```python
from build123d import *

# Parameters (mm, degrees)
SKETCH1_W                    = 104.78
SKETCH1_H                    = 53.63
BOSS_EXTRUDE1_DEPTH          = 6.35
F_0_257_DIAMETER_HOLE1_D     = 6.5278
F_30_0_1285_DIAMETER_HOLE1_D = 3.2639
FILLET1_R                    = 5


with BuildPart() as part:
    # Sketch1 → Boss-Extrude1 (new body)
    with BuildSketch(Plane(origin=(0, 0, 0), x_dir=(1, 0, 0), z_dir=(0, 1, 0))):
        with Locations((52.39, 26.815)):
            Rectangle(SKETCH1_W, SKETCH1_H)
    extrude(amount=BOSS_EXTRUDE1_DEPTH)

    # F (0.257) Diameter Hole1 (through all)
    with Locations(Plane(origin=(0, 0, 0), x_dir=(-1, 0, 0), z_dir=(0, -1, 0))):
        with Locations((-52.39, 26.815)):
            Hole(F_0_257_DIAMETER_HOLE1_D / 2)

    # #30 (0.1285) Diameter Hole1 (through all)
    with Locations(Plane(origin=(0, 0, 0), x_dir=(-1, 0, 0), z_dir=(0, -1, 0))):
        with Locations((-9.525, 7.765), (-9.525, 45.865), (-95.25, 45.865), (-95.25, 7.765)):
            Hole(F_30_0_1285_DIAMETER_HOLE1_D / 2)

    # Fillet1
    fillet1_edges = [part.edges().sort_by_distance(p)[0] for p in [
        (0, 3.175, -53.63),
        (104.78, 3.175, -53.63),
        (104.78, 3.175, 0),
        (0, 3.175, 0),
    ]]
    fillet(fillet1_edges, radius=FILLET1_R)


solid = part.part
```
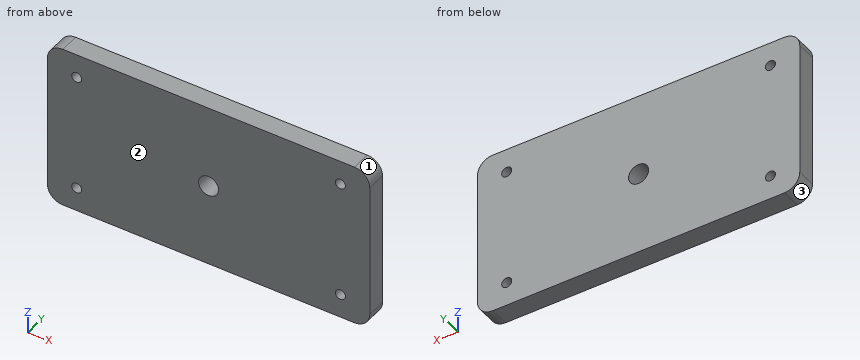
Check sheet for the modelled part. Datum: model origin and axes. Units: mm. Face numbers are marked on the shaded views. Give positions to 0.01 mm unless a question says otherwise; leave off trailing zeros. Order: outer loops, then holes, each group sorted by start corner. A loop starts at its lowest first (then second) coordinate and runs counter-clockwise, first axis right, second up. Notation, with made-up numbers: M -33.75,25.5 L 24.25,25.5 A3 cw 24.25,29.5 Z; hole C 38.5,2.25 d9. An arc over 180 degrees is marked long. Answer in a Markdown table with one row per item. Add a question column.
Q1. Release check for a two-part mould opening along X. For the marked faces 1, 2 and 3 record: released by +X, released by -X, zero draft, split by the parting line, or undercut.
Q2. Thickness scan on L1, parallel to Z at x = 95.25, y = 4.5; L2, parallel to Z at x = 10, y = 4.25; L3, parallel to X at y = 5.5, z = -47. Record the ranges inside material, lowest first.
Q3. Sectioned sample at B-B, the plane x = 52.39. Record the boundary of the cut face in (y, z).
Q4. Gauge pin test, flat end, axial feed: pin 1 Ø2 at (x, z) = (9.525, -45.865) entering from -Y. Record the tip position at first contact, or that the pin passes through.
Q5. Sectioned sample at C-C, the plane y = 4. Record the boundary of the cut face in (x, z) (3 decimals), and give its area (3 significant figures).
Q6. Sectioned sample at A-A, the plane x = 95.25. Record the boundary of the cut face in (y, z).
Verdict:
| question | item | result |
|---|---|---|
| 1 | face 1 | released by +X |
| 1 | face 2 | zero draft |
| 1 | face 3 | released by -X |
| 2 | L1 | -53.63 to -47.5, -44.23 to -9.4, -6.13 to 0 |
| 2 | L2 | -53.63 to -47.43, -44.3 to -9.33, -6.2 to 0 |
| 2 | L3 | 0 to 8.35, 10.7 to 94.08, 96.42 to 104.78 |
| 3 | outline | M 0,-53.63 L 6.35,-53.63 L 6.35,-30.08 L 0,-30.08 Z; M 0,-23.55 L 6.35,-23.55 L 6.35,0 L 0,0 Z |
| 4 | pin 1 | through |
| 5 | outline | M 0,-48.63 A5 ccw 5,-53.63 L 99.78,-53.63 A5 ccw 104.78,-48.63 L 104.78,-5 A5 ccw 99.78,0 L 5,0 A5 ccw 0,-5 Z; hole C 9.525,-45.865 d3.264; hole C 9.525,-7.765 d3.264; hole C 52.39,-26.815 d6.528; hole C 95.25,-45.865 d3.264; hole C 95.25,-7.765 d3.264 |
| 5 | area | 5,530 mm² |
| 6 | outline | M 0,-53.63 L 6.35,-53.63 L 6.35,-47.5 L 0,-47.5 Z; M 0,-44.23 L 6.35,-44.23 L 6.35,-9.4 L 0,-9.4 Z; M 0,-6.13 L 6.35,-6.13 L 6.35,0 L 0,0 Z |
